Here's how the part is built. I have some questions about the finished solid (model axes, mm). A direction names the side the tool comes from. Coordinates: 2 decimals unless noted, no trailing zeros. Write each loop counter-clockwise with the first axis right and the second up, starting at its lowest first coordinate (ties: lowest second). Pieces come first, ordered by that corner, then holes. Notation, with made-up numbers: M 86,-3.75 L 103,-3.75 A19 cw 103,1.25 Z; hole C -23,-20.5 d9. An arc over 180 degrees is marked long. Use a Markdown table: item, result.
```python
from build123d import *

# Parameters (mm, degrees)
F0_R     = 17.5
F0_R_2   = 15.75
F1_DEPTH = 7
F0_R_3   = 2.5
F2_DEPTH = 3
F3_SIZE  = 1


# Not quite as in the source:
# - a feature names something its author has since deleted; it is built from what else it names


with BuildPart() as f1:
    # F0 (on Top) → F1 (new body)
    with BuildSketch(Plane.XY):
        Circle(F0_R)
        Circle(F0_R_2, mode=Mode.SUBTRACT)
    extrude(amount=F1_DEPTH)

    # F0 (on Top) → F2 (join)
    with BuildSketch(Plane.XY):
        Circle(F0_R_2)
        Circle(F0_R_3, mode=Mode.SUBTRACT)
    extrude(amount=F2_DEPTH)

    # F3
    f3_edges = [f1.edges().sort_by_distance(p)[0] for p in [
        (-15.75, 0, 7),
    ]]
    chamfer(f3_edges, length=F3_SIZE)


solid = f1.part
```
1. Suppose I cut it at C-C on z = 4. Write out the boundary of the cut face in (x, y).
Answers follow:
| item | result |
|---|---|
| outline | C 0,0 d35; hole C 0,0 d31.5 |
2. Suppose I cut it at A-A on x = 0. Write out the boundary of the cut face in (y, z), and give its area (3 significant figures).
Answers follow:
| item | result |
|---|---|
| outline | M -17.5,0 L -2.5,0 L -2.5,3 L -15.75,3 L -15.75,6 L -16.75,7 L -17.5,7 Z; M 2.5,0 L 17.5,0 L 17.5,7 L 16.75,7 L 15.75,6 L 15.75,3 L 2.5,3 Z |
| area | 103 mm2 |
3. Will these pins go through, and if not, where does the flat tip stop? pin 1 Ø8 at (x, y) = (0, 0) entering from +Z; pin 2 Ø2 at (y, z) = (10, 5) entering from -X.
Answers follow:
| item | result |
|---|---|
| pin 1 | stops at z = 3 |
| pin 2 | stops at x = -15.01 |
4. We'd pull the mould along X, two halves only. Please class faces 3 (the face through (-13.887, -10.648, 3.451)), 4 (the face through (0, -4, 0)), 5 (the face through (-2.05, 15.616, 4.479)): +X half, -X half, draft (parallel to the pull), parting line (faces both ways), or undercut.
Answers follow:
| item | result |
|---|---|
| face 3 | parting line |
| face 4 | draft |
| face 5 | undercut |
5. Suppose I cut it at D-D on z = 2. Write out the boundary of the cut face in (x, y), and give its area (3 significant figures).
Answers follow:
| item | result |
|---|---|
| outline | C 0,0 d35; hole C 0,0 d5 |
| area | 942 mm2 |
6. I need wall thicknesses on probe 1 along Y at (x, z) = (0, 1); probe 2 along Y at (x, z) = (0, 5.2); probe 3 along Z at (x, y) = (2.5, 8). Which ranges of each line are inside material? Lowest first, please.
Answers follow:
| item | result |
|---|---|
| probe 1 | y = -17.5 to -2.5, 2.5 to 17.5 |
| probe 2 | y = -17.5 to -15.75, 15.75 to 17.5 |
| probe 3 | z = 0 to 3 |
7. Which directions (+Z, -Z, +X, -X, +Y, -Y) give clear straight access to the entire face, cutting with the end or side of a thin tool? Please do faces 1 (the face through (3, 0, 3)), 2 (the face through (0, -17, 7)).
Answers follow:
| item | result |
|---|---|
| face 1 | +Z |
| face 2 | +Z, +X, -X, +Y, -Y |
